```python
from build123d import *

# Parameters (mm, degrees)
EXTRUDE_2_DEPTH     = 6.5
CUT_EXTRUDE_1_DEPTH = 3
SKETCH_4_R          = 0.5
CUT_EXTRUDE_2_DEPTH = 5
SKETCH_5_W          = 10.662315839
SKETCH_5_H          = 14.474999285
CUT_EXTRUDE_3_DEPTH = 15
SKETCH_6_W          = 18
SKETCH_6_H          = 6.5630452
SKETCH_6_W_2        = 18.4
SKETCH_6_H_2        = 6.601696298
CUT_EXTRUDE_4_DEPTH = 4.5
SKETCH_8_W          = 13.913437684
SKETCH_8_H          = 10.074999285
CUT_EXTRUDE_5_DEPTH = 3.2
SKETCH_9_R          = 1.65
CUT_EXTRUDE_6_DEPTH = 23
CHAMFER_2_SIZE      = 1
FILLET_1_R          = 1
SKETCH_20_W         = 43.816957605
SKETCH_20_H         = 2
SKETCH_20_W_2       = 44.126249409
SKETCH_20_W_3       = 44.36192542
CUT_EXTRUDE_7_DEPTH = 1.5
FILLET_2_R          = 1
SKETCH_21_W         = 13.231285314
SKETCH_21_H         = 4.572576543
SKETCH_21_W_2       = 12.647552139
SKETCH_21_H_2       = 6.080553912
CUT_EXTRUDE_8_DEPTH = 1.5
CHAMFER_3_SIZE      = 1


with BuildPart() as part:
    # Эскиз2 → Бобышка-Вытянуть2 (new body)
    with BuildSketch(Plane.XY):
        Polygon((-1.450000048, 28.424999237), (-3.400000095, 26.475000381), (-3.400000095, -1.450000048), (-1.399999976, -3.450000048), (46.449998499, -3.450000048), (48.474998474, -1.424999952), (48.474998474, 26.350000381), (46.400001526, 28.424999237), align=None)
    extrude(amount=EXTRUDE_2_DEPTH)

    # Эскиз3 → Вырез-Вытянуть1 (cut)
    with BuildSketch(Plane(origin=(0, 0, 0), x_dir=(-1, 0, 0), z_dir=(0, 0, -1))):
        with BuildLine():
            Line((-45.474998474, -2.450000048), (-4.599999905, -2.450000048))
            ThreePointArc((-4.599999905, -2.450000048), (-3.185786342, -1.86421361), (-2.599999905, -0.450000048))
            Line((-2.599999905, -0.450000048), (-2.599999905, 0.549999952))
            ThreePointArc((-2.599999905, 0.549999952), (-2.014213467, 1.964213515), (-0.599999905, 2.549999952))
            Line((-0.599999905, 2.549999952), (0.400000095, 2.549999952))
            ThreePointArc((0.400000095, 2.549999952), (1.814213658, 3.13578639), (2.400000095, 4.549999952))
            Line((2.400000095, 4.549999952), (2.400000095, 20.424999237))
            ThreePointArc((2.400000095, 20.424999237), (1.814213658, 21.839212799), (0.400000095, 22.424999237))
            Line((0.400000095, 22.424999237), (-0.599999905, 22.424999237))
            ThreePointArc((-0.599999905, 22.424999237), (-2.014213467, 23.010785675), (-2.599999905, 24.424999237))
            Line((-2.599999905, 24.424999237), (-2.599999905, 25.424999237))
            ThreePointArc((-2.599999905, 25.424999237), (-3.185786342, 26.839212799), (-4.599999905, 27.424999237))
            Line((-4.599999905, 27.424999237), (-45.474998474, 27.424999237))
            ThreePointArc((-45.474998474, 27.424999237), (-46.889212036, 26.839212799), (-47.474998474, 25.424999237))
            Line((-47.474998474, 25.424999237), (-47.474998474, -0.450000048))
            ThreePointArc((-47.474998474, -0.450000048), (-46.889212036, -1.86421361), (-45.474998474, -2.450000048))
        make_face()
    extrude(amount=-CUT_EXTRUDE_1_DEPTH, mode=Mode.SUBTRACT)

    # Эскиз4 → Вырез-Вытянуть2 (cut)
    with BuildSketch(Plane(origin=(0, 0, 0), x_dir=(-1, 0, 0), z_dir=(0, 0, -1))):
        with Locations((0, 25)):
            Circle(SKETCH_4_R)
        Circle(SKETCH_4_R)
    extrude(amount=-CUT_EXTRUDE_2_DEPTH, mode=Mode.SUBTRACT)

    # Эскиз5 → Вырез-Вытянуть3 (cut)
    with BuildSketch(Plane(origin=(0, 0, 0), x_dir=(-1, 0, 0), z_dir=(0, 0, -1))):
        with Locations((-45.306156394, 12.787499595)):
            Rectangle(SKETCH_5_W, SKETCH_5_H)
    extrude(amount=-CUT_EXTRUDE_3_DEPTH, mode=Mode.SUBTRACT)

    # Эскиз6 → Вырез-Вытянуть4 (cut)
    with BuildSketch(Plane(origin=(0, 0, 0), x_dir=(-1, 0, 0), z_dir=(0, 0, -1))):
        with Locations((-31.974998474, 25.706521837)):
            Rectangle(SKETCH_6_W, SKETCH_6_H)
        with Locations((-31.874998474, -0.750848197)):
            Rectangle(SKETCH_6_W_2, SKETCH_6_H_2)
    extrude(amount=-CUT_EXTRUDE_4_DEPTH, mode=Mode.SUBTRACT)

    # Эскиз8 → Вырез-Вытянуть5 (cut)
    with BuildSketch(Plane(origin=(0, 0, 0), x_dir=(-1, 0, 0), z_dir=(0, 0, -1))):
        with Locations((-1.643281063, 12.587499595)):
            Rectangle(SKETCH_8_W, SKETCH_8_H)
    extrude(amount=-CUT_EXTRUDE_5_DEPTH, mode=Mode.SUBTRACT)

    # Эскиз9 → Вырез-Вытянуть6 (cut)
    with BuildSketch(Plane(origin=(0, 0, 3), x_dir=(-1, 0, 0), z_dir=(0, 0, -1))):
        with Locations((-30.274998474, 13.724999237)):
            Circle(SKETCH_9_R)
        with Locations((-0.599999905, 19.724999237)):
            Circle(SKETCH_9_R)
        with Locations(Location((-0.599999905, 6.049999952, 0), (0, 0, 65.380022671))):
            Circle(SKETCH_9_R)
    extrude(amount=-CUT_EXTRUDE_6_DEPTH, mode=Mode.SUBTRACT)

    # Фаска2
    chamfer_2_edges = [part.edges().sort_by_distance(p)[0] for p in [
        (-3.400000095, 12.512500167, 6.5),
        (-2.400000036, -2.450000048, 6.5),
        (22.524999262, -3.450000048, 6.5),
        (47.462498487, -2.4375, 6.5),
        (48.474998474, 2.0625, 6.5),
        (47.4375, 27.387499809, 6.5),
        (22.475000739, 28.424999237, 6.5),
        (48.474998474, 23.187499809, 6.5),
        (-2.425000072, 27.449999809, 6.5),
    ]]
    chamfer(chamfer_2_edges, length=CHAMFER_2_SIZE)

    # Скругление1
    fillet_1_edges = [part.edges().sort_by_distance(p)[0] for p in [
        (40.974998474, 22.424999237, 3.75),
        (22.974998474, 22.424999237, 3.75),
        (22.674998474, 2.549999952, 3.75),
        (41.074998474, 2.549999952, 3.75),
        (8.599999905, 17.624999237, 3.1),
        (8.599999905, 7.549999952, 3.1),
        (39.974998474, 5.549999952, 4.75),
        (39.974998474, 20.024999237, 4.75),
    ]]
    fillet(fillet_1_edges, radius=FILLET_1_R)

    # Эскиз20 → Вырез-Вытянуть7 (cut)
    with BuildSketch(Plane.XY.offset(6.5)):
        with Locations((13.066519672, 23.424999237)):
            Rectangle(SKETCH_20_W, SKETCH_20_H)
        with Locations((13.066519672, 13.424999237)):
            Rectangle(SKETCH_20_W, SKETCH_20_H)
        with Locations((12.91187377, 1.424999237)):
            Rectangle(SKETCH_20_W_2, SKETCH_20_H)
        with Locations((13.066519672, 7.424999237)):
            Rectangle(SKETCH_20_W, SKETCH_20_H)
        with Locations((12.794035764, 18.424999237)):
            Rectangle(SKETCH_20_W_3, SKETCH_20_H)
    extrude(amount=-CUT_EXTRUDE_7_DEPTH, mode=Mode.SUBTRACT)

    # Скругление2
    fillet_2_edges = [part.edges().sort_by_distance(p)[0] for p in [
        (34.974998474, 0.424999237, 5.75),
        (34.974998474, 6.424999237, 5.75),
        (34.974998474, 12.424999237, 5.75),
        (34.974998474, 17.424999237, 5.75),
        (34.974998474, 2.424999237, 5.75),
        (34.974998474, 8.424999237, 5.75),
        (34.974998474, 14.424999237, 5.75),
        (34.974998474, 19.424999237, 5.75),
        (34.974998474, 22.424999237, 5.75),
        (34.974998474, 24.424999237, 5.75),
    ]]
    fillet(fillet_2_edges, radius=FILLET_2_R - 0.0001)  # a hair under: the kernel refuses the full size

    # Эскиз21 → Вырез-Вытянуть8 (cut)
    with BuildSketch(Plane.XY.offset(6.5)):
        with Locations((-0.015642752, 20.906096965)):
            Rectangle(SKETCH_21_W, SKETCH_21_H)
        with Locations((0.276223836, 4.43995697)):
            Rectangle(SKETCH_21_W_2, SKETCH_21_H_2)
    extrude(amount=-CUT_EXTRUDE_8_DEPTH, mode=Mode.SUBTRACT)

    # Фаска3
    chamfer_3_edges = [part.edges().sort_by_distance(p)[0] for p in [
        (6.599999905, 20.924999237, 6.5),
        (6.599999905, 4.424999237, 6.5),
    ]]
    chamfer(chamfer_3_edges, length=CHAMFER_3_SIZE)


solid = part.part
```
Input: part model. Units: mm. Frame: model coordinates. A direction names the side the tool comes from. Round coordinates to 2 decimals unless told otherwise and drop trailing zeros. Loops run counter-clockwise (first coordinate to the right, second up) from the corner with the lowest first, then second, coordinate; pieces in that order, holes last. Notation, with made-up numbers: M 36,-28 L 68,-28 A20 ccw 68,6 Z; hole C 25.25,79.5 d9. An arc over 180 degrees is marked long. Answer in a Markdown table with one row per item. Add a question column.
1. Ray query, probe 1 along Y at (x, z) = (14, 5.25) (3 decimals); probe 2 along X at (y, z) = (0, 2.75) (3 decimals); probe 3 along Y at (x, z) = (0, 1.7) (3 decimals). Return the intervals inside material, ascending.
2. Contact query for flat-ended pins moving along their axis: pin 1 (2 mm diameter, centred on x = 7.5, y = 23.5, fed in from -Z); pin 2 (1 mm diameter, centred on x = 20.5, y = 13, fed in from +Z); pin 3 (0.8 mm diameter, centred on x = 25, z = 6, fed in from +Y) (3 decimals). Output: stop coordinate, or through.
3. Set-up query: faces 1 (the face through (22.81, 27.918, 6.007)), 2 (the face through (0, 2.55, 1)), 3 (the face through (34.674, 12.71, 5.74)). Return all of +Z, -Z, +X, -X, +Y, -Y with unobstructed straight access to the full face (end or side cutting, diameter ignored); none if empty.
4. Section B-B (z = 1.75). Give the number of separate pieces and of enclosed holes in the cut face, and give its area (3 significant figures).
5. Section A-A (y = 11.5). Output: boundary loops of the cut face in (x, z) (3 decimals).
6. Mould query, pull axis X, two halves, no side actions, for faces 4 (the face through (47.1, -2.103, 5.993)), 5 (the face through (40.975, 26.4, 3.2)), 6 (the face through (34.674, 8.14, 5.74)), 7 (the face through (41.075, -1.5, 3.2)). Classes: released by +X, released by -X, zero draft, split by the parting line, or undercut.
Values follow:
| question | item | result |
|---|---|---|
| 1 | probe 1 | -3.45 to 0.425, 2.425 to 6.425, 8.425 to 12.425, 14.425 to 17.425, 19.425 to 22.425, 24.425 to 28.425 |
| 1 | probe 2 | -3.4 to -0.5, 0.5 to 2.6, 47.475 to 48.475 |
| 1 | probe 3 | -3.45 to -0.5, 0.5 to 2.55, 22.425 to 24.5, 25.5 to 28.425 |
| 2 | pin 1 | z = 3 |
| 2 | pin 2 | z = 5 |
| 2 | pin 3 | y = 28.325 |
| 3 | face 1 | +Z, +X, -X, +Y |
| 3 | face 2 | -Z |
| 3 | face 3 | +Z, -X |
| 4 | separate pieces | 4 |
| 4 | enclosed holes | 2 |
| 4 | area | 146 mm^2 |
| 5 | outline | M -3.4,3.2 L 8.6,3.2 L 8.6,3 L 39.975,3 L 39.975,6.5 L -2.4,6.5 L -3.4,5.5 Z |
| 6 | face 4 | released by +X |
| 6 | face 5 | undercut |
| 6 | face 6 | released by -X |
| 6 | face 7 | undercut |
